Geometry: see drawing. Coordinates: mm, zero at the bounding-box minimum. Give positions to 0.01 mm unless a question says otherwise; leave off trailing zeros. Write each loop counter-clockwise with the first axis right and the second up, starting at its lowest first coordinate (ties: lowest second). Pieces come first, ordered by that corner, then holes. Notation, with made-up numbers: M 36,12.25 L 58,12.25 A30 ccw 58,38.25 Z; hole C -38,45 d4. An arc over 180 degrees is marked long. Answer as a JSON object with one key per item and string values. Group by question number.
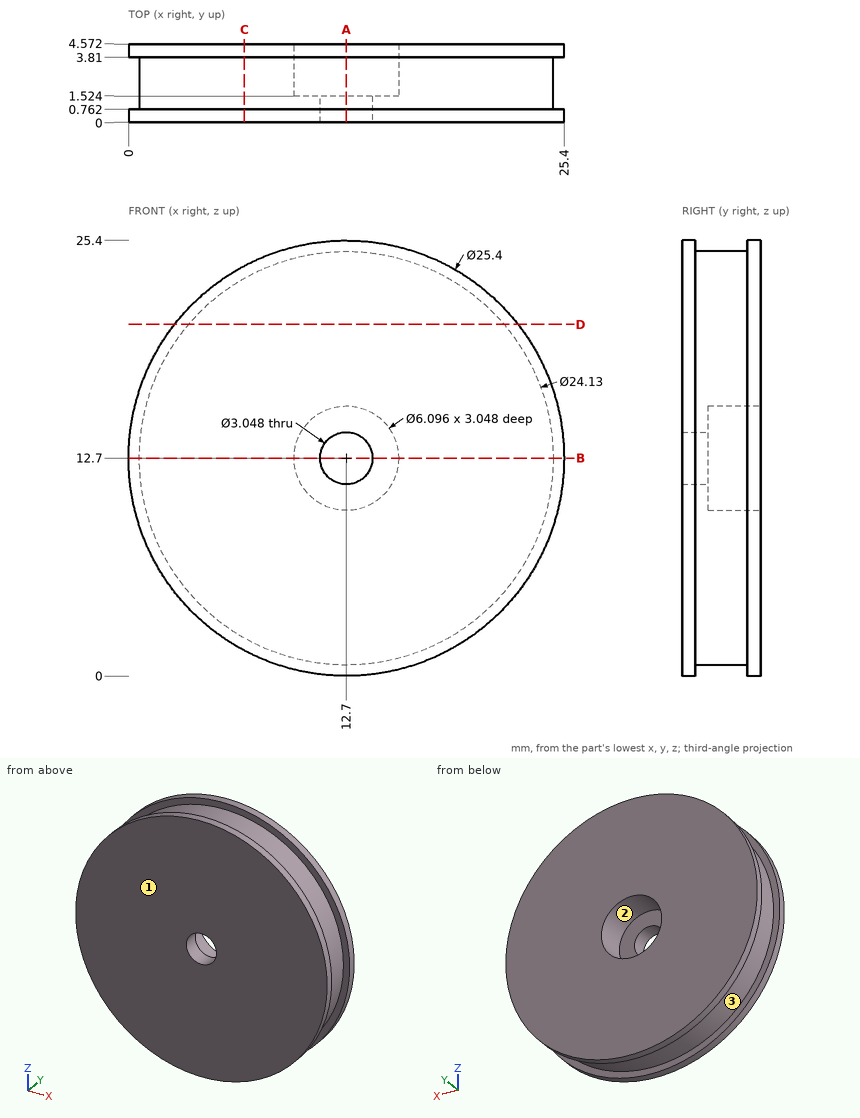
(1) Ray query, L1, parallel to X at y = 3.4, z = 12.7 (3 decimals); L2, parallel to Z at x = 12.7, y = 0.95 (3 decimals); L3, parallel to Y at x = 3, z = 4.75. Return the intervals inside material, ascending. Write a range as [from, to].
(2) Section B-B, the plane z = 12.7. Return loops of the section in (x, y) (3 decimals), plus the area to 3 significant figures.
(3) Section A-A, the plane x = 12.7. Return loops of the section in (y, z) (3 decimals).
(4) Contact query for flat-ended pins moving along their axis: pin 1 Ø1 at (y, z) = (1, 5) entering from -X; pin 2 Ø4 at (x, z) = (12.7, 12.7) entering from +Y; pin 3 Ø1 at (x, y) = (15, 1) entering from -Z. Output: stop coordinate, or through.
(5) Pull-direction query (Z, two-part tool) for the marked faces 1, 2 and 3; classes: pulls with the +Z half, pulls with the -Z half, needs draft (parallel to the pull), parting line crosses it, or undercut.
(6) Section D-D, the plane z = 20.5. Return loops of the section in (x, y).
(7) Section C-C, the plane x = 6.75. Return loops of the section in (y, z), plus the area to 3 significant figures.
Reported:
{
 "1": {"L1": "x = [0.635, 9.652], [15.748, 24.765]", "L2": "z = [0.635, 11.176], [14.224, 24.765]", "L3": "y = [0, 0.76], [3.81, 4.57]"},
 "2": {"outline": "M 0,0 L 11.176,0 L 11.176,1.524 L 9.652,1.524 L 9.652,4.572 L 0,4.572 L 0,3.81 L 0.635,3.81 L 0.635,0.762 L 0,0.762 Z; M 14.224,0 L 25.4,0 L 25.4,0.762 L 24.765,0.762 L 24.765,3.81 L 25.4,3.81 L 25.4,4.572 L 15.748,4.572 L 15.748,1.524 L 14.224,1.524 Z", "area": "89.0 mm2"},
 "3": {"outline": "M 0,0 L 0.762,0 L 0.762,0.635 L 3.81,0.635 L 3.81,0 L 4.572,0 L 4.572,9.652 L 1.524,9.652 L 1.524,11.176 L 0,11.176 Z; M 0,14.224 L 1.524,14.224 L 1.524,15.748 L 4.572,15.748 L 4.572,25.4 L 3.81,25.4 L 3.81,24.765 L 0.762,24.765 L 0.762,25.4 L 0,25.4 Z"},
 "4": {"pin 1": "stops at x = 2.28", "pin 2": "stops at y = 1.52", "pin 3": "stops at z = 0.14"},
 "5": {"face 1": "needs draft", "face 2": "undercut", "face 3": "parting line crosses it"},
 "6": {"outline": "M 2.68,0 L 22.72,0 L 22.72,0.76 L 21.9,0.76 L 21.9,3.81 L 22.72,3.81 L 22.72,4.57 L 2.68,4.57 L 2.68,3.81 L 3.5,3.81 L 3.5,0.76 L 2.68,0.76 Z"},
 "7": {"outline": "M 0,1.48 L 0.76,1.48 L 0.76,2.2 L 3.81,2.2 L 3.81,1.48 L 4.57,1.48 L 4.57,23.92 L 3.81,23.92 L 3.81,23.2 L 0.76,23.2 L 0.76,23.92 L 0,23.92 Z", "area": "98.2 mm2"}
}
